Study the drawing (mm; zero at the part's minimum x, y, z) and answer. Give positions to 0.01 mm unless a question says otherwise; leave off trailing zeros. Order: outer loops, then holes, each group sorted by start corner. A loop starts at its lowest first (then second) coordinate and runs counter-clockwise, first axis right, second up.
Item 1: A cutting plane is placed at A-A (x = 85). Write down the section's boundary in (y, z).
Item 2: Given pin 1 Ø1.5 at (x, y) = (1.5, 1.5) entering from +Z; pin 2 Ø1.5 at (x, y) = (77.5, 1.5) entering from -Z; pin 3 Ø0.9 at (y, z) = (1, 1) entering from -X, each flat-ended and moving along its own axis, determine where each tip first touches the part or whether it passes through.
Item 3: A cutting plane is placed at B-B (z = 24). Write down the section's boundary in (x, y).
Item 4: Find the intervals of material crossed by line 1 along Z through (x, y) = (85, 1); line 2 along X through (y, z) = (1.8, 20.5); line 3 along Z through (x, y) = (77.5, 0.65), in increasing order.
Item 5: A cutting plane is placed at C-C (x = 26.5). Write down the section's boundary in (y, z).
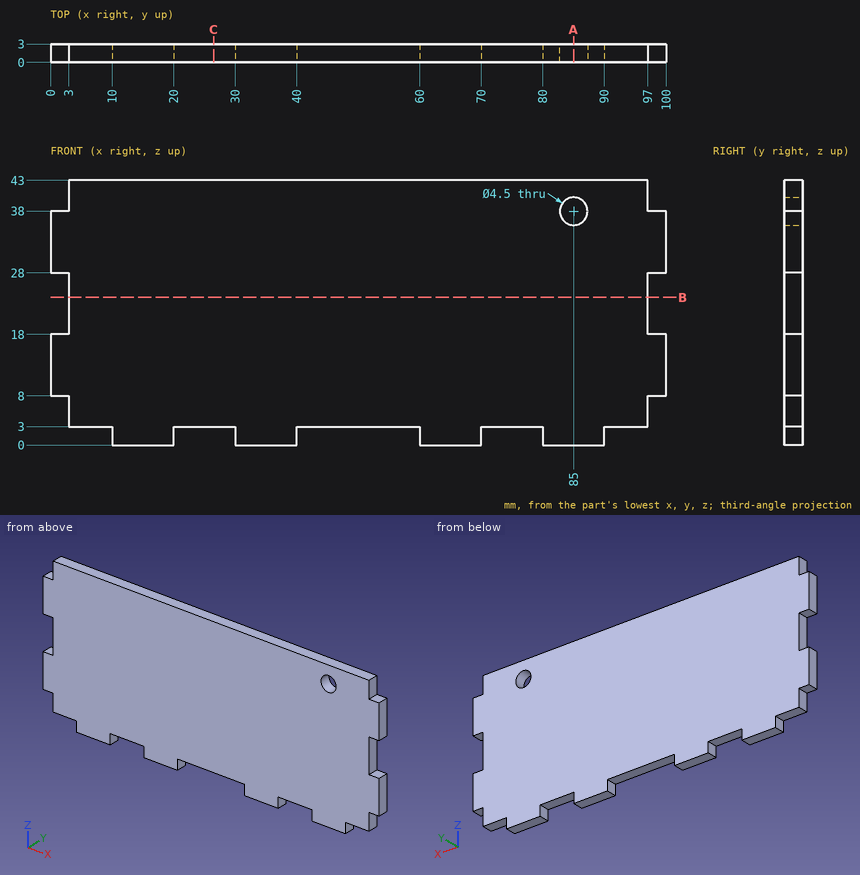
Response values:
1. outline: (0, 0) - (3, 0) - (3, 35.75) - (0, 35.75) - close; (0, 40.25) - (3, 40.25) - (3, 43) - (0, 43) - close
2. pin 1: stops at z = 38
2. pin 2: stops at z = 3
2. pin 3: stops at x = 10
3. outline: (3, 0) - (97, 0) - (97, 3) - (3, 3) - close
4. line 1: z = 0 to 35.75, 40.25 to 43
4. line 2: x = 3 to 97
4. line 3: z = 3 to 43
5. outline: (0, 3) - (3, 3) - (3, 43) - (0, 43) - close
